```python
from build123d import *

# Parameters (mm, degrees)
SKETCH1_W           = 34
SKETCH1_H           = 60
SKETCH1_R           = 3.39
SKETCH1_R_2         = 0.75
BOSS_EXTRUDE1_DEPTH = 3
CHAMFER1_SIZE       = 1.3
SKETCH2_R           = 0.8
CUT_EXTRUDE1_DEPTH  = 3


with BuildPart() as part:
    # Sketch1 → Boss-Extrude1 (new body)
    with BuildSketch(Plane.XY):
        Rectangle(SKETCH1_W, SKETCH1_H)
        Circle(SKETCH1_R, mode=Mode.SUBTRACT)
        with Locations((-15, -27.5)):
            Circle(SKETCH1_R_2, mode=Mode.SUBTRACT)
        with Locations(Location((-15, 27.5, 0), (0, 0, 180))):
            Circle(SKETCH1_R_2, mode=Mode.SUBTRACT)
        with Locations((15, 27.5)):
            Circle(SKETCH1_R_2, mode=Mode.SUBTRACT)
    extrude(amount=BOSS_EXTRUDE1_DEPTH)

    # Chamfer1
    # the kernel refuses this chamfer: 1.3 mm, written as the material it takes off along each edge
    with BuildSketch(Plane(origin=(-15, -27.5, 3), x_dir=(1, 0, 0), z_dir=(0, -1, 0))) as chamfer1_piece_1:
        Polygon((0.75, -CHAMFER1_SIZE), (0.75 + CHAMFER1_SIZE, 0), (0.75, 0), align=None)
    revolve(axis=Axis((-15, -27.5, 3), (0, 0, 1)), mode=Mode.SUBTRACT)
    with BuildSketch(Plane(origin=(-15, 27.5, 3), x_dir=(-1, 0, 0), z_dir=(0, 1, 0))) as chamfer1_piece_2:
        Polygon((0.75, -CHAMFER1_SIZE), (0.75 + CHAMFER1_SIZE, 0), (0.75, 0), align=None)
    revolve(axis=Axis((-15, 27.5, 3), (0, 0, 1)), mode=Mode.SUBTRACT)
    with BuildSketch(Plane(origin=(15, 27.5, 3), x_dir=(1, 0, 0), z_dir=(0, -1, 0))) as chamfer1_piece_3:
        Polygon((0.75, -CHAMFER1_SIZE), (0.75 + CHAMFER1_SIZE, 0), (0.75, 0), align=None)
    revolve(axis=Axis((15, 27.5, 3), (0, 0, 1)), mode=Mode.SUBTRACT)

    # Sketch2 → Cut-Extrude1 (cut)
    with BuildSketch(Plane(origin=(17, 0, 0), x_dir=(0, 0, -1), z_dir=(1, 0, 0))):
        with Locations((-1.5, -27)):
            Circle(SKETCH2_R)
    extrude(amount=-CUT_EXTRUDE1_DEPTH, mode=Mode.SUBTRACT)


solid = part.part
```
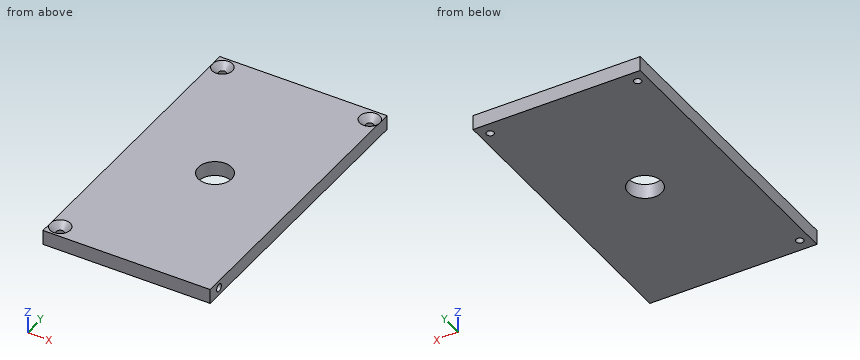
Check sheet for the modelled part. Datum: model origin and axes. Units: mm. Round coordinates to 2 decimals unless told otherwise and drop trailing zeros. Order: outer loops, then holes, each group sorted by start corner. A loop starts at its lowest first (then second) coordinate and runs counter-clockwise, first axis right, second up. Notation, with made-up numbers: (0, 83) - (50, 83) arc R30 cw to (50, 117) - close; hole circle Ø2 at (37, 10). An arc over 180 degrees is marked (long way). Write item = value, one per line.
Q1. Go/stop test with flat-tipped pins: pin 1 (0.5 mm diameter, centred on y = -27, z = 1.5, fed in from +X); pin 2 (0.9 mm diameter, centred on x = 15, y = 27.5, fed in from +Z); pin 3 (2.5 mm diameter, centred on x = -15, y = -27.5, fed in from +Z). Record where each tip stops, or that it passes through.
Computed:
pin_1 = 14
pin_2 = through
pin_3 = 2.2
Q2. Thickness scan on line 1 along Y through (x, z) = (-15, 1.3); line 2 along Y through (x, z) = (-14.5, 1.65); line 3 along Y through (x, z) = (0, 1.2). Record the ranges inside material, lowest first.
Computed:
line_1 = -30 to -28.25, -26.75 to 26.75, 28.25 to 30
line_2 = -30 to -28.06, -26.94 to 26.94, 28.06 to 30
line_3 = -30 to -3.39, 3.39 to 30
Q3. Section check B-B (y = 0). Record the boundary of the cut face in (x, z), and give its area (3 significant figures).
Computed:
outline = (-17, 0) - (-3.39, 0) - (-3.39, 3) - (-17, 3) - close; (3.39, 0) - (17, 0) - (17, 3) - (3.39, 3) - close
area = 81.7 mm^2
Q4. Section check C-C (z = 1.2). Record the boundary of the cut face in (x, y), and give its area (3 significant figures).
Computed:
outline = (-17, -30) - (17, -30) - (17, -27.74) - (14, -27.74) - (14, -26.26) - (17, -26.26) - (17, 30) - (-17, 30) - close; hole circle Ø1.5 at (-15, -27.5); hole circle Ø1.5 at (-15, 27.5); hole circle Ø6.78 at (0, 0); hole circle Ø1.5 at (15, 27.5)
area = 1,990 mm^2
Q5. Section check A-A (x = 15). Record the boundary of the cut face in (y, z), and give its area (3 significant figures).
Computed:
outline = (-30, 0) - (26.75, 0) - (26.75, 1.7) - (25.45, 3) - (-30, 3) - close; (28.25, 0) - (30, 0) - (30, 3) - (29.55, 3) - (28.25, 1.7) - close; hole circle Ø1.6 at (-27, 1.5)
area = 172 mm^2
